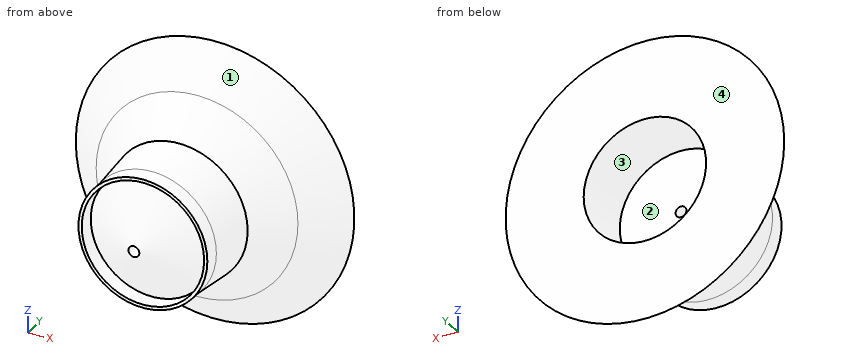
Autodesk Fusion 360 part; units mm, degrees
sketch "Sketch1" plane through (0, 0, 0) normal (0, 1, 0) x (1, 0, 0)
  circle A0 centre (0, 0) radius 18.5
  circle A1 centre (0, 0) radius 20
  dimension "d1" = 37
  dimension "d2" = 1.5
extrude "Extrude1" add sketch "Sketch1" along normal blind 15 draft 5 and the other way blind 5
sketch "Sketch2" plane through (0, 15, 0) normal (0, 1, 0) x (-1, 0, 0)
  circle A0 centre (0, 0) radius 17.1877
  circle A1 centre (0, 0) radius 21.3123
  circle A2 centre (0, 0) radius 17.1877
  circle A3 centre (0, 0) radius 21.3123
extrude "Extrude2" add sketch "Sketch2" along normal blind 10 draft 45
sketch "Sketch3" plane through (0, 25, 0) normal (0, 1, 0) x (-1, 0, 0)
  circle A0 centre (0, 0) radius 7.1877
  circle A1 centre (0, 0) radius 31.3123
  circle A2 centre (0, 0) radius 12.1877
  circle A3 centre (0, 0) radius 26.3123
extrude "Extrude3" add sketch "Sketch3" along normal blind 10 draft 50 contours A1 | A3
sketch "Sketch4" plane through (0, 25, 0) normal (0, 1, 0) x (-1, 0, 0)
  circle A0 centre (0, 0) radius 12.1877
  circle A1 centre (0, 0) radius 7.1877
  circle A2 centre (0, 0) radius 7.1877
extrude "Extrude4" cut sketch "Sketch4" along normal blind 60 contours A1 A2
sketch "Sketch5" plane through (0, 35, 0) normal (0, 1, 0) x (-1, 0, 0)
  circle A0 centre (0, 0) radius 7.1877
  circle A1 centre (0, 0) radius 43.2299
  circle A2 centre (0, 0) radius 35
extrude "Extrude5" cut sketch "Sketch5" against normal blind 20 draft -50 contours A2
ref_plane "WorkPlane1" through (0, 15, 0) normal (0, 1, 0) x (0, 0, 1)
sketch "Sketch6" plane through (0, 15, 0) normal (0, 1, 0) x (1, 0, 0)
  circle A0 centre (0, 0) radius 19
  dimension "d16" = 38
extrude "Extrude6" cut sketch "Sketch6" along normal blind -70 and the other way blind -65
sketch "Sketch7" plane through (0, 15, 0) normal (0, 1, 0) x (1, 0, 0)
  circle A0 centre (0, 0) radius 19
extrude "Extrude7" add sketch "Sketch7" against normal blind 15
sketch "Sketch8" plane through (0, 0, 0) normal (0, -1, 0) x (1, 0, 0)
  circle A0 centre (0, 0) radius 19
  circle A1 centre (0, 0) radius 19
extrude "Extrude8" add sketch "Sketch8" along normal blind 10 draft -60
sketch "Sketch9" plane through (0, -10, 0) normal (0, -1, 0) x (1, 0, 0)
  circle A0 centre (0, 0) radius 1.6795
  circle A1 centre (0, 0) radius 1.6795
  dimension "d27" = 3.359
extrude "Extrude9" cut sketch "Sketch9" against normal blind 60
Verification items for the finished model (mm, model axes). Face numbers are marked on the shaded views. Round coordinates to 2 decimals unless told otherwise and drop trailing zeros. Loops run counter-clockwise (first coordinate to the right, second up) from the corner with the lowest first, then second, coordinate; pieces in that order, holes last. Notation, with made-up numbers: (-29, -11) - (24, -11) arc R28 ccw to (24, 27) - close; hole circle Ø7 at (38, 40.25). An arc over 180 degrees is marked (long way). Use a Markdown table: item, result. Add a question column.
1. Section check D-D, the plane y = 13. Record the boundary of the cut face in (x, z), plus the area to 3 significant figures.
2. Section check A-A, the plane x = 0. Record the boundary of the cut face in (y, z), plus the area to 3 significant figures.
3. Section check C-C, the plane y = 4. Record the boundary of the cut face in (x, z).
4. Release check for a two-part mould opening along X. For the marked faces 1, 2, 3 and 4 record: released by +X, released by -X, zero draft, split by the parting line, or undercut.
5. Thickness scan on probe 1 along X at (y, z) = (-1, 2.5); probe 2 along Z at (x, y) = (-16.5, -2); probe 3 along X at (y, z) = (15.5, 17.5). Record the ranges inside material, lowest first. Write a range as [from, to].
6. Gauge pin test, flat ends, axial feed: pin 1 (1 mm diameter, centred on x = -23, z = 14.5, fed in from -Y); pin 2 (8 mm diameter, centred on x = -7.5, y = 21.5, fed in from -Z); pin 3 (6 mm diameter, centred on x = -3.5, y = 10.5, fed in from +Z). Record the tip position at first contact, or that the pin passes through.
7. Section check B-B, the plane z = 0. Record the boundary of the cut face in (x, y), plus the area to 3 significant figures.
Checks:
| question | item | result |
|---|---|---|
| 1 | outline | circle Ø42.27 at (0, 0); hole circle Ø3.36 at (0, 0) |
| 1 | area | 1,390 mm^2 |
| 2 | outline | (-10, -1.68) - (0, -19) - (-5, -19) - (-5, -20) - (0, -20) - (15, -21.31) - (25, -31.31) - (35, -43.23) - (35, -19) - (15, -19) - (15, -1.68) - close; (-10, 1.68) - (15, 1.68) - (15, 19) - (35, 19) - (35, 43.23) - (25, 31.31) - (15, 21.31) - (0, 20) - (-5, 20) - (-5, 19) - (0, 19) - close |
| 2 | area | 1,260 mm^2 |
| 3 | outline | circle Ø40.7 at (0, 0); hole circle Ø3.36 at (0, 0) |
| 4 | face 1 | split by the parting line |
| 4 | face 2 | undercut |
| 4 | face 3 | undercut |
| 4 | face 4 | zero draft |
| 5 | probe 1 | x = [-19.84, -18.83], [-17.09, 17.09], [18.83, 19.84] |
| 5 | probe 2 | z = [-11.3, -9.42], [9.42, 11.3] |
| 5 | probe 3 | x = [-13.02, -7.4], [7.4, 13.02] |
| 6 | pin 1 | stops at y = 20.38 |
| 6 | pin 2 | stops at z = -31.1 |
| 6 | pin 3 | stops at z = 21.06 |
| 7 | outline | (-43.23, 35) - (-31.31, 25) - (-21.31, 15) - (-20, 0) - (-20, -5) - (-19, -5) - (-19, 0) - (-1.68, -10) - (-1.68, 15) - (-19, 15) - (-19, 35) - close; (1.68, -10) - (19, 0) - (19, -5) - (20, -5) - (20, 0) - (21.31, 15) - (31.31, 25) - (43.23, 35) - (19, 35) - (19, 15) - (1.68, 15) - close |
| 7 | area | 1,260 mm^2 |
